from build123d import *

# Parameters (mm, degrees)
F0_W     = 203.2
F0_H     = 12.7
F1_DEPTH = 38.1
F2_W     = 12.7
F2_H     = 44.917874
F3_DEPTH = 25.4
F4_R     = 12.7
F5_SIZE  = 10.16
F6_R     = 6.35
F7_DEPTH = 228.6
F8_R     = 7.314346
F9_DEPTH = 25.4


with BuildPart() as f1:
    # F0 (on Right) → F1 (new body)
    with BuildSketch(Plane.YZ):
        with Locations((-79.141063, 31.75)):
            Rectangle(F0_W, F0_H)
        with Locations((-79.141063, 19.05)):
            Rectangle(F0_W, F0_H)
        with Locations((-79.141063, 6.35)):
            Rectangle(F0_W, F0_H)
    extrude(amount=F1_DEPTH)

    # F2 (on face) → F3 (join)
    with BuildSketch(Plane(origin=(0, 0, 0), x_dir=(1, 0, 0), z_dir=(0, 0, -1))):
        with Locations((19.05, 0)):
            Rectangle(F2_W, F2_H)
    extrude(amount=F3_DEPTH)

    # F4
    f4_edges = [f1.edges().sort_by_distance(p)[0] for p in [
        (38.1, -79.141063, 38.1),
        (0, -79.141063, 38.1),
    ]]
    fillet(f4_edges, radius=F4_R)

    # F5
    f5_edges = [f1.edges().sort_by_distance(p)[0] for p in [
        (38.1, -79.141063, 0),
        (0, -79.141063, 0),
    ]]
    chamfer(f5_edges, length=F5_SIZE)

    # F6 (on face) → F7 (cut)
    with BuildSketch(Plane.XZ.offset(180.741063)):
        with Locations((19.05, 17.78)):
            Circle(F6_R)
    extrude(amount=-F7_DEPTH, mode=Mode.SUBTRACT)

    # F8 (on face) → F9 (cut)
    with BuildSketch(Plane.YZ.offset(25.4)):
        with Locations((0, -12.215126)):
            Circle(F8_R)
    extrude(amount=-F9_DEPTH, mode=Mode.SUBTRACT)


solid = f1.part
Could you check a few things on this model? Use its own coordinates, in mm. A direction names the side the tool comes from. Round coordinates to 2 decimals unless told otherwise and drop trailing zeros. Write each loop counter-clockwise with the first axis right and the second up, starting at its lowest first coordinate (ties: lowest second). Pieces come first, ordered by that corner, then holes. Notation, with made-up numbers: (-8, 48) -> (39, 48) arc R31 cw to (39, 86) -> close; hole circle Ø10 at (-13, 57.25). An arc over 180 degrees is marked (long way). Use a Markdown table: item, result.
1. If we section it at C-C (y = -46): List the corners of the cut face in (x, z) for me.
Answer key:
| item | result |
|---|---|
| outline | (0, 10.16) -> (10.16, 0) -> (27.94, 0) -> (38.1, 10.16) -> (38.1, 25.4) arc R12.7 ccw to (25.4, 38.1) -> (12.7, 38.1) arc R12.7 ccw to (0, 25.4) -> close; hole circle Ø12.7 at (19.05, 17.78) |
2. We'd pull the mould along Z, two halves only. Please class faces 1 (the face through (23, -180.741, 24)), 2 (the face through (3.82, -77.72, 34.48)), 3 (the face through (22.464, -80.563, 23.134)): +Z half, -Z half, draft (parallel to the pull), parting line (faces both ways), or undercut.
Answer key:
| item | result |
|---|---|
| face 1 | draft |
| face 2 | +Z half |
| face 3 | undercut |
3. For pin 1 Ø7.5 at (x, z) = (19.05, 17.78) entering from -Y; pin 2 Ø9 at (x, y) = (18, -41) entering from -Z; pin 3 Ø4 at (y, z) = (-118, 5) entering from -X; pin 4 Ø20.5 at (y, z) = (-2, -13) entering from +X, each with a flat end and sliding along its axis, tell me the tip position at first contact or that it passes through.
Answer key:
| item | result |
|---|---|
| pin 1 | passes through |
| pin 2 | stops at z = 0 |
| pin 3 | stops at x = 3.16 |
| pin 4 | stops at x = 25.4 |
4. Please list where these lines run through material, in increasing order: probe 1 along Z at (x, y) = (18.5, 0); probe 2 along Z at (x, y) = (17, 0); probe 3 along Z at (x, y) = (25.5, -95).
Answer key:
| item | result |
|---|---|
| probe 1 | z = -25.4 to -19.53, -4.9 to 11.45, 24.11 to 38.1 |
| probe 2 | z = -25.4 to -19.53, -4.9 to 11.77, 23.79 to 38.1 |
| probe 3 | z = 0 to 38.1 |
5. If we section it at D-D (z = 17.78): List the corners of the cut face in (x, y) for me.
Answer key:
| item | result |
|---|---|
| outline | (0, -180.74) -> (12.7, -180.74) -> (12.7, 22.46) -> (0, 22.46) -> close; (25.4, -180.74) -> (38.1, -180.74) -> (38.1, 22.46) -> (25.4, 22.46) -> close |
6. Which directions (+Z, -Z, +X, -X, +Y, -Y) give clear straight access to the entire face, cutting with the end or side of a thin tool? Please do faces 4 (the face through (12.7, 5, -18)), 5 (the face through (19, -22.459, -13)), 6 (the face through (19, -81, 38.1)), 7 (the face through (25.4, 5, -18)), 8 (the face through (19, 0, -25.4)).
Answer key:
| item | result |
|---|---|
| face 4 | -Z, -X, +Y, -Y |
| face 5 | -Z, +X, -X, -Y |
| face 6 | +Z, +X, -X, +Y, -Y |
| face 7 | -Z, +X, +Y, -Y |
| face 8 | -Z, +X, -X, +Y, -Y |
7. If we section it at B-B (x = 19.05): List the corners of the cut face in (y, z) for me, then the cut area to 3 significant figures.
Answer key:
| item | result |
|---|---|
| outline | (-180.74, 0) -> (-22.46, 0) -> (-22.46, -25.4) -> (22.46, -25.4) -> (22.46, 11.43) -> (-180.74, 11.43) -> close; (-180.74, 24.13) -> (22.46, 24.13) -> (22.46, 38.1) -> (-180.74, 38.1) -> close; hole circle Ø14.63 at (0, -12.22) |
| area | 6,130 mm^2 |
8. If we section it at A-A (y = 0): List the corners of the cut face in (x, z) for me, then the cut area to 3 significant figures.
Answer key:
| item | result |
|---|---|
| outline | (0, 10.16) -> (10.16, 0) -> (12.7, 0) -> (12.7, -4.9) -> (25.4, -4.9) -> (25.4, 0) -> (27.94, 0) -> (38.1, 10.16) -> (38.1, 25.4) arc R12.7 ccw to (25.4, 38.1) -> (12.7, 38.1) arc R12.7 ccw to (0, 25.4) -> close; (12.7, -25.4) -> (25.4, -25.4) -> (25.4, -19.53) -> (12.7, -19.53) -> close; hole circle Ø12.7 at (19.05, 17.78) |
| area | 1,290 mm^2 |
